Input: part model. Units: mm. Frame: model coordinates. A direction names the side the tool comes from. Coordinates: 2 decimals unless noted, no trailing zeros. Loops run counter-clockwise (first coordinate to the right, second up) from the corner with the lowest first, then second, coordinate; pieces in that order, holes last. Notation, with made-up numbers: M 83.25,21.25 L 134.25,21.25 A30 ccw 134.25,59.25 Z; hole C 1,65 d7. An arc over 180 degrees is marked long. Use a Markdown table: item, result. Add a question column.
1. Section D-D on x = 72.5. Output: boundary loops of the cut face in (y, z).
2. Section A-A on x = -42. Output: boundary loops of the cut face in (y, z).
3. Line query: L1, parallel to Z at x = -10, y = 17.25; L2, parallel to Z at x = 41.5, y = 4.25; L3, parallel to Z at x = 61.5, y = 12.75. Output: solid intervals per line, ascending. Write a range as [from, to].
4. Set-up query: faces 5 (the cylindrical face through (-44.777, 10.14, 59.96)), 6 (the flat face through (-70, 15, 100)), 7 (the flat face through (0, 5, 16)), 8 (the flat face through (85, 10, 100)). Return all of +Z, -Z, +X, -X, +Y, -Y with unobstructed straight access to the full face (end or side cutting, diameter ignored); none if empty.
5. Draft query along X for faces 1 (the flat face through (16, 5, 0)), 2 (the flat face through (85, 15, 120)), 3 (the flat face through (0, 5, -16)), 4 (the flat face through (100, 10, 21)). Return one class per face: +X half, -X half, draft (parallel to the pull), parting line (faces both ways), or undercut.
6. Section B-B on y = 4.75. State how many separate pieces and enclosed holes the cut face has, then the cut area to 3 significant figures.
7. Pin query (flat end, axial travel): pin 1 (24 mm diameter, centred on x = 79.5, z = 98.5, fed in from -Y). Return the tip coordinate at first contact, or that it passes through.
8. Section C-C on z = 83. Output: boundary loops of the cut face in (x, y).
Autodesk Inventor part; units mm, degrees
ref_plane "YZ Plane" through (0, 0, 0) normal (1, 0, 0) x (0, 1, 0)
ref_plane "XZ Plane" through (0, 0, 0) normal (0, 1, 0) x (-1, 0, 0)
ref_plane "XY Plane" through (0, 0, 0) normal (0, 0, 1) x (1, 0, 0)
sketch "Boceto1" plane through (0, 0, 0) normal (0, 1, 0) x (-1, 0, 0)
  line L0 (100, 80) -> (-100, 80)
  line L1 (-100, 80) -> (-100, -80)
  line L2 (-100, -80) -> (100, -80)
  line L3 (100, -80) -> (100, 80)
  line L4 (100, 80) -> (-100, -80) construction
  line L5 (-100, 80) -> (100, -80) construction
  point P0 (0, 0)
  dimension "d0" = 200
  dimension "d1" = 160
extrude "Extrusión1" add sketch "Boceto1" along normal blind 20
sketch "Boceto2" plane through (0, 20, 0) normal (0, 1, 0) x (1, 0, 0)
  circle A0 centre (-90, -57.83) radius 3.5
  line L0 (-100, -65.43) -> (-32, -65.43)
  line L1 (-32, -65.43) -> (-32, 14.57)
  line L2 (-32, 14.57) -> (-100, 14.57)
  line L3 (-100, 14.57) -> (-100, -65.43)
  line L4 (-66, -65.43) -> (-66, -8.508)
  circle A1 centre (-66, -57.83) radius 3.5
  circle A2 centre (-42, -57.83) radius 3.5
  line L5 (-32, -25.43) -> (-48.2072, -25.43)
  circle A3 centre (-42, 6.97) radius 3.5
  circle A4 centre (-66, 6.97) radius 3.5
  circle A5 centre (-90, 6.97) radius 3.5
  circle A6 centre (-60, 55) radius 5
  line L6 (-100, 80) -> (-100, -80)
  line L7 (0, 0) -> (0, -20.5185)
  circle A7 centre (90, -57.83) radius 3.5
  circle A8 centre (66, -57.83) radius 3.5
  circle A9 centre (42, -57.83) radius 3.5
  line L8 (100, -65.43) -> (32, -65.43)
  line L9 (66, -65.43) -> (66, -8.508)
  line L10 (32, -25.43) -> (48.2072, -25.43)
  circle A10 centre (90, 6.97) radius 3.5
  line L11 (100, 14.57) -> (100, -65.43)
  circle A11 centre (66, 6.97) radius 3.5
  line L12 (32, 14.57) -> (100, 14.57)
  line L13 (32, -65.43) -> (32, 14.57)
  circle A12 centre (42, 6.97) radius 3.5
  circle A13 centre (60, 55) radius 5
  line L14 (100, 80) -> (100, -80)
  dimension "d4" = 7
  dimension "d5" = 68
  dimension "d6" = 80
  dimension "d7" = 7.6
  dimension "d8" = 10
  dimension "d9" = 7
  dimension "d10" = 24
  dimension "d11" = 10
  dimension "d16" = 0
  dimension "d19" = 40
extrude "Extrusión2" cut sketch "Boceto2" against normal blind 20 contours A0 | A1 L4 | L4 A1 | A2 | A3 | A4 | A5 | A7 | A8 L9 | L9 A8 | A9 | A10 | A11 | A12
sketch "Boceto3" plane through (-100, 0, 80) normal (0, 0, 1) x (1, 0, 0)
  line L0 (0, 20) -> (30, 20)
  line L1 (30, 20) -> (30, 10)
  line L2 (30, 10) -> (0, 10)
  line L3 (0, 10) -> (0, 20)
  line L4 (100, 0) -> (100, 11.6249)
  line L5 (200, 20) -> (170, 20)
  line L6 (170, 20) -> (170, 10)
  line L7 (170, 10) -> (200, 10)
  line L8 (200, 10) -> (200, 20)
  dimension "d22" = 30
  dimension "d23" = 10
extrude "Extrusión3" add sketch "Boceto3" along normal blind 40
sketch "Boceto4" plane through (0, 20, 0) normal (0, 1, 0) x (1, 0, 0)
  line L0 (-60, 60) -> (-60, 50)
  line L1 (-70, 50) -> (-70, 60)
  line L2 (-60, 50) -> (-70, 60) construction
  line L3 (-70, 50) -> (-60, 60) construction
  line L4 (-60, 50) -> (-70, 50)
  circle A0 centre (-68.25, 51.75) radius 1.75
  line L5 (-70, 60) -> (-60, 60)
  circle A1 centre (-61.75, 58.25) radius 1.75
  line L6 (100, 80) -> (-100, 80)
  line L7 (0, 80) -> (0, 60)
  line L8 (60, 60) -> (60, 50)
  circle A2 centre (61.75, 58.25) radius 1.75
  line L9 (70, 60) -> (60, 60)
  line L10 (70, 50) -> (70, 60)
  line L11 (60, 50) -> (70, 60) construction
  line L12 (70, 50) -> (60, 60) construction
  line L13 (60, 50) -> (70, 50)
  circle A3 centre (68.25, 51.75) radius 1.75
  line L14 (-100, 80) -> (-100, -120)
  line L15 (100, 80) -> (100, -120)
  point P0 (0, 0)
  point P1 (-70.0286, 64.971)
  point P2 (-65, 50)
  point P3 (70.0286, 64.971)
  point P4 (65, 50)
  dimension "d26" = 1.75
  dimension "d27" = 8.25
  dimension "d28" = 20
  dimension "d29" = 10
  dimension "d30" = 10
  dimension "d31" = 1.75
  dimension "d32" = 1.75
  dimension "d33" = 1.75
  dimension "d58" = 30
  dimension "d59" = 30
extrude "Extrusión4" cut sketch "Boceto4" against normal blind 40 contours A1 | A0 | A2 | A3
sketch "Boceto5" plane through (0, 20, 0) normal (0, 1, 0) x (1, 0, 0)
  line L0 (-100, -80) -> (-100, -120)
  line L1 (-70.0001, -120) -> (-70.0001, -80)
  line L2 (-55.1959, -79.9497) -> (-70.0001, -80)
  line L3 (-70.0001, -80) -> (-100, -80)
  line L4 (-100, -120) -> (-70.0001, -120)
  line L5 (-64.3507, -80) -> (-74.3507, -80)
  circle A0 centre (-81.75, -108.25) radius 1.75
  circle A1 centre (-88.25, -101.75) radius 1.75
  line L6 (-70.0001, -80) -> (70.0001, -80)
  line L7 (0, -80) -> (0, -101.75)
  circle A2 centre (81.75, -108.25) radius 1.75
  circle A3 centre (88.25, -101.75) radius 1.75
  line L8 (-70, -80) -> (70, -80)
  line L9 (-100, 80) -> (-100, -120)
  point P0 (0, 0)
  point P1 (-81.75, -101.75)
  point P2 (-63.4459, -118.25)
  point P3 (81.75, -101.75)
  dimension "d36" = 11.7499
  dimension "d37" = 40
  dimension "d38" = 29.9999
  dimension "d39" = 21.75
  dimension "d40" = 11.75
  dimension "d41" = 28.3003
  dimension "d42" = 11.7499
  dimension "d43" = 0
  dimension "d44" = 0
hole "Agujero1" at (-88.25, 20, 101.75) at (-81.75, 20, 108.25) at (81.75, 20, 108.25) at (88.25, 20, 101.75) direction (0, -1, 0) diameter 3.5 end through all
ref_plane "Plano de trabajo1" through (100, 0, 0) normal (0, 0, -1) x (-1, 0, 0)
ref_plane "Plano de trabajo2" through (0, 0, -80) normal (-1, 0, 0) x (0, 0, 1)
sketch "Boceto6" plane through (0, 0, 0) normal (0, -1, 0) x (1, 0, 0)
  circle A0 centre (10, -10) radius 1.75
  line L0 (6.803, 0) -> (14.6069, 0)
  line L1 (0, 0) -> (0, -4.8284)
  line L2 (0, 0) -> (20.0354, 0)
  circle A1 centre (10, 10) radius 1.75
  line L3 (0, 0) -> (0, 4.8284)
  circle A2 centre (-10, 10) radius 1.75
  circle A3 centre (-10, -10) radius 1.75
  dimension "d63" = 3.5
  dimension "d64" = 10
  dimension "d65" = 10
hole "Agujero2" at (10, 0, 10) at (-10, 0, 10) at (-10, 0, -10) at (10, 0, -10) direction (0, 1, 0) diameter 3.5 end through all
sketch "Boceto7" plane through (0, 0, 0) normal (0, -1, 0) x (1, 0, 0)
  line L0 (-16, 16) -> (16, 16)
  line L1 (16, 16) -> (16, -16)
  line L2 (16, -16) -> (-16, -16)
  line L3 (-16, -16) -> (-16, 16)
  line L4 (-16, 16) -> (16, -16) construction
  line L5 (16, 16) -> (-16, -16) construction
  point P0 (0, 0)
  point P1 (0, 0)
  point P2 (0, 0)
  dimension "d73" = 32
  dimension "d74" = 32
extrude "Extrusión5" cut sketch "Boceto7" against normal blind 10
sketch "Boceto8" plane through (0, 20, 0) normal (0, 1, 0) x (1, 0, 0)
  line L0 (-15, -60) -> (15, -60)
  circle A0 centre (10, -65) radius 1.75
  line L1 (-10, -65) -> (10, -65)
  line L2 (15, -60) -> (15, -70)
  circle A1 centre (-10, -65) radius 1.75
  line L3 (-15, -70) -> (15, -60) construction
  line L4 (-15, -60) -> (15, -70) construction
  line L5 (-15, -70) -> (-15, -60)
  line L6 (15, -70) -> (-15, -70)
  point P0 (0, 0)
  point P1 (0, -69.1269)
  point P2 (-15, -67.1661)
  point P3 (0, -69.1269)
  point P4 (15, -65)
  dimension "d77" = 10
  dimension "d78" = 30
  dimension "d79" = 5
  dimension "d80" = 5
  dimension "d81" = 5
  dimension "d82" = 5
hole "Agujero3" at (-10, 20, 65) at (10, 20, 65) direction (0, -1, 0) diameter 3.5 end through all
properties part number "base_back_20"
Answers below:
| question | item | result |
|---|---|---|
| 1 | outline | M 0,-80 L 20,-80 L 20,120 L 10,120 L 10,80 L 0,80 Z |
| 2 | outline | M 0,-80 L 20,-80 L 20,-10.47 L 0,-10.47 Z; M 0,-3.47 L 20,-3.47 L 20,54.33 L 0,54.33 Z; M 0,61.33 L 20,61.33 L 20,80 L 0,80 Z |
| 3 | L1 | z = [-80, -11.75], [-8.25, 8.25], [11.75, 63.25], [66.75, 80] |
| 3 | L2 | z = [-80, -10.43], [-3.51, 54.37], [61.29, 80] |
| 3 | L3 | z = [-80, -59.98], [-56.52, 80] |
| 4 | face 5 | +Y, -Y |
| 4 | face 6 | +Z, +Y, -Y |
| 4 | face 7 | -Y |
| 4 | face 8 | +Z, +X, -X, -Y |
| 5 | face 1 | undercut |
| 5 | face 2 | draft |
| 5 | face 3 | undercut |
| 5 | face 4 | +X half |
| 6 | separate pieces | 1 |
| 6 | enclosed holes | 19 |
| 6 | area | 30,500 mm² |
| 7 | pin 1 | stops at y = 10 |
| 8 | outline | M -100,10 L -70,10 L -70,20 L -100,20 Z; M 70,10 L 100,10 L 100,20 L 70,20 Z |
